Geometry check sheet. Reference: the model listing, model coordinates, mm. Face numbers are marked on the shaded views. A direction names the side the tool comes from. Give positions to 0.01 mm unless a question says otherwise; leave off trailing zeros. Order: outer loops, then holes, each group sorted by start corner. A loop starts at its lowest first (then second) coordinate and runs counter-clockwise, first axis right, second up. Notation, with made-up numbers: M -17,84.5 L -5,84.5 A22 ccw -5,107.5 Z; hole C 84.25,46.25 d1. An arc over 180 degrees is marked long. One line per question, with ' | ' between items. Start each with the question number.
from build123d import *
from OCP.BRepFilletAPI import BRepFilletAPI_MakeChamfer

# Parameters (mm, degrees)
SKETCH1_W           = 1.85
SKETCH1_H           = 38.85
SKETCH1_H_2         = 6.15
SKETCH1_W_2         = 44.85
SKETCH1_H_3         = 1.85
SKETCH1_W_3         = 0.15
BOSS_EXTRUDE1_DEPTH = 3
SKETCH1_4_W         = 120
SKETCH1_4_H         = 30
SKETCH1_4_W_2       = 30
SKETCH1_4_H_2       = 120
BOSS_EXTRUDE3_DEPTH = 4
CHAMFER1_SIZE       = 2.5
CHAMFER1_SIZE2      = 9.330127019
SKETCH4_W           = 8.5
SKETCH4_H           = 30
SKETCH4_W_2         = 30
SKETCH4_H_2         = 8.5
CUT_EXTRUDE1_DEPTH  = 1.5
BOSS_EXTRUDE4_DEPTH = 35
CHAMFER2_SIZE       = 6
BOSS_EXTRUDE5_DEPTH = 3
CHAMFER3_SIZE       = 2
CHAMFER3_SIZE2      = 5.494954839
BOSS_EXTRUDE6_DEPTH = 2.5


with BuildPart() as part:
    # Sketch1 → Boss-Extrude1 (new body)
    with BuildSketch(Plane(origin=(0, 0, 0), x_dir=(-1, 0, 0), z_dir=(0, 0, -1))):
        with Locations((14.075, 40.575)):
            Rectangle(SKETCH1_W, SKETCH1_H)
        with Locations((14.075, 18.075)):
            Rectangle(SKETCH1_W, SKETCH1_H_2)
        with Locations((37.575, 14.075)):
            Rectangle(SKETCH1_W_2, SKETCH1_H_3)
        with Locations((14.075, 14.075)):
            Rectangle(SKETCH1_W, SKETCH1_H_3)
        with Locations((14.075, -14.075)):
            Rectangle(SKETCH1_W, SKETCH1_H_3)
        with Locations((14.075, -18.075)):
            Rectangle(SKETCH1_W, SKETCH1_H_2)
        with Locations((37.575, -14.075)):
            Rectangle(SKETCH1_W_2, SKETCH1_H_3)
        with Locations((14.075, -40.575)):
            Rectangle(SKETCH1_W, SKETCH1_H)
        with Locations((-14.075, -14.075)):
            Rectangle(SKETCH1_W, SKETCH1_H_3)
        with Locations((-14.075, -18.075)):
            Rectangle(SKETCH1_W, SKETCH1_H_2)
        with Locations((-37.575, -14.075)):
            Rectangle(SKETCH1_W_2, SKETCH1_H_3)
        with Locations((-15.075, -14.075)):
            Rectangle(SKETCH1_W_3, SKETCH1_H_3)
        with Locations((15.075, -14.075)):
            Rectangle(SKETCH1_W_3, SKETCH1_H_3)
        with Locations((15.075, 14.075)):
            Rectangle(SKETCH1_W_3, SKETCH1_H_3)
        with Locations((-37.575, 14.075)):
            Rectangle(SKETCH1_W_2, SKETCH1_H_3)
        with Locations((-15.075, 14.075)):
            Rectangle(SKETCH1_W_3, SKETCH1_H_3)
        with Locations((-14.075, 18.075)):
            Rectangle(SKETCH1_W, SKETCH1_H_2)
        with Locations((-14.075, 14.075)):
            Rectangle(SKETCH1_W, SKETCH1_H_3)
        with Locations((-14.075, 40.575)):
            Rectangle(SKETCH1_W, SKETCH1_H)
        with Locations((-14.075, -40.575)):
            Rectangle(SKETCH1_W, SKETCH1_H)
    extrude(amount=-BOSS_EXTRUDE1_DEPTH)

    # Sketch1<4> → Boss-Extrude3 (add)
    with BuildSketch(Plane(origin=(0, 0, 0), x_dir=(-1, 0, 0), z_dir=(0, 0, -1))):
        Rectangle(SKETCH1_4_W, SKETCH1_4_H)
        Rectangle(SKETCH1_4_W_2, SKETCH1_4_H_2)
    extrude(amount=BOSS_EXTRUDE3_DEPTH)

    # Chamfer1: one chamfer whose edges measure the first distance from different faces: ONE call of the kernel's chamfer builder (chamfer() names one face for all edges)
    chamfer1_edges_1 = [part.edges().sort_by_distance(p)[0] for p in [
        (60, 0, -4),
    ]]
    chamfer1_side_1 = [part.faces().sort_by_distance(p)[0] for p in [
        (60, 0, -1.703661327),
    ]]
    chamfer1_edges_2 = [part.edges().sort_by_distance(p)[0] for p in [
        (0, 60, -4),
    ]]
    chamfer1_side_2 = [part.faces().sort_by_distance(p)[0] for p in [
        (0, 60, -1.703661327),
    ]]
    chamfer1_edges_3 = [part.edges().sort_by_distance(p)[0] for p in [
        (0, -60, -4),
    ]]
    chamfer1_side_3 = [part.faces().sort_by_distance(p)[0] for p in [
        (0, -60, -1.703661327),
    ]]
    chamfer1_edges_4 = [part.edges().sort_by_distance(p)[0] for p in [
        (-60, 0, -4),
    ]]
    chamfer1_side_4 = [part.faces().sort_by_distance(p)[0] for p in [
        (-60, 0, -1.703661327),
    ]]
    chamfer1 = BRepFilletAPI_MakeChamfer(part.part.solid().wrapped)
    for e in chamfer1_edges_1:
        chamfer1.Add(CHAMFER1_SIZE, CHAMFER1_SIZE2, e.wrapped, chamfer1_side_1[0].wrapped)  # the first distance lies on this face
    for e in chamfer1_edges_2:
        chamfer1.Add(CHAMFER1_SIZE, CHAMFER1_SIZE2, e.wrapped, chamfer1_side_2[0].wrapped)  # the first distance lies on this face
    for e in chamfer1_edges_3:
        chamfer1.Add(CHAMFER1_SIZE, CHAMFER1_SIZE2, e.wrapped, chamfer1_side_3[0].wrapped)  # the first distance lies on this face
    for e in chamfer1_edges_4:
        chamfer1.Add(CHAMFER1_SIZE, CHAMFER1_SIZE2, e.wrapped, chamfer1_side_4[0].wrapped)  # the first distance lies on this face
    add(Compound.cast(chamfer1.Shape()), mode=Mode.REPLACE)

    # Sketch4 → Cut-Extrude1 (cut)
    with BuildSketch(Plane(origin=(0, 0, -4), x_dir=(-1, 0, 0), z_dir=(0, 0, -1))):
        with Locations((-41.419872981, 0)):
            Rectangle(SKETCH4_W, SKETCH4_H)
        with Locations((-29.919872981, 0)):
            Rectangle(SKETCH4_W, SKETCH4_H)
        with Locations((0, 41.419872981)):
            Rectangle(SKETCH4_W_2, SKETCH4_H_2)
        with Locations((0, 29.919872981)):
            Rectangle(SKETCH4_W_2, SKETCH4_H_2)
        with Locations((29.919872981, 0)):
            Rectangle(SKETCH4_W, SKETCH4_H)
        with Locations((41.419872981, 0)):
            Rectangle(SKETCH4_W, SKETCH4_H)
        with Locations((0, -29.919872981)):
            Rectangle(SKETCH4_W_2, SKETCH4_H_2)
        with Locations((0, -41.419872981)):
            Rectangle(SKETCH4_W_2, SKETCH4_H_2)
    extrude(amount=-CUT_EXTRUDE1_DEPTH, mode=Mode.SUBTRACT)

    # Sketch5 → Boss-Extrude4 (add)
    with BuildSketch(Plane(origin=(0, 0, -4), x_dir=(-1, 0, 0), z_dir=(0, 0, -1))):
        Polygon((-7.424621202, 3.181980515), (-3.181980515, 7.424621202), (7.424621202, -3.181980515), (3.181980515, -7.424621202), align=None)
    extrude(amount=BOSS_EXTRUDE4_DEPTH)

    # Chamfer2
    chamfer2_edges = [part.edges().sort_by_distance(p)[0] for p in [
        (-2.121320344, 2.121320344, -39),
    ]]
    chamfer(chamfer2_edges, length=CHAMFER2_SIZE - 0.0001)  # a hair under: the kernel refuses the full size

    # Sketch6 → Boss-Extrude5 (add)
    with BuildSketch(Plane(origin=(-12.727922061, 12.727922061, -18), x_dir=(-0.8660254037844379, -0.28867513459481464, 0.4082482904638634), z_dir=(-0.5000000000000013, 0.5000000000000013, -0.7071067811865458))):
        Polygon((-23.270152556, -19.918584287), (-11.723147173, -3.588652668), (0.524301541, -12.248906706), (-11.022703843, -28.578838325), align=None)
    extrude(amount=BOSS_EXTRUDE5_DEPTH)

    # Chamfer3
    chamfer3_edges = [part.edges().sort_by_distance(p)[0] for p in [
        (-9.378679656, 9.378679656, -26.97918472),
    ]]
    chamfer3_side = [part.faces().sort_by_distance(p)[0] for p in [
        (-8.628679656, 8.628679656, -25.918524548),
    ]]
    chamfer(chamfer3_edges, length=CHAMFER3_SIZE, length2=CHAMFER3_SIZE2, reference=chamfer3_side[0])

    # Sketch8 → Boss-Extrude6 (add)
    with BuildSketch(Plane(origin=(-11.477922061, 11.477922061, -16.232233047), x_dir=(0.8660254037844378, 0.28867513459481475, -0.4082482904638635), z_dir=(0.5000000000000016, -0.5000000000000013, 0.7071067811865456))):
        Polygon((6.123724357, -21.650635095), (18.371173071, -12.990381057), (9.885891697, -0.990381057), (-2.361557017, -9.650635095), align=None)
    extrude(amount=BOSS_EXTRUDE6_DEPTH)


solid = part.part
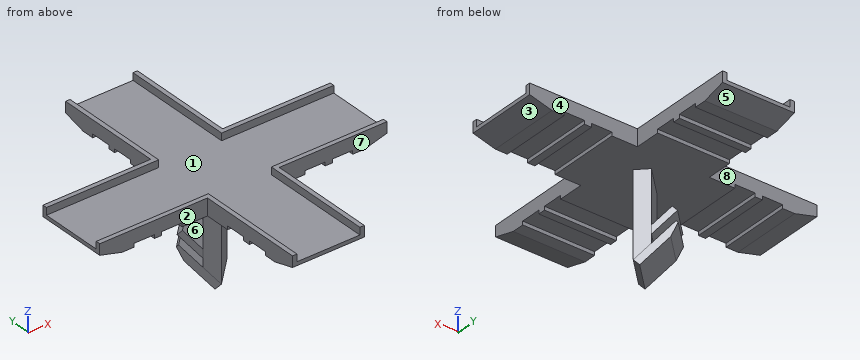
Item 1: Cross-section at B-B, the plane y = 22.5. Record the cut outline in (x, z), plus the area to 3 significant figures.
Item 2: Depth check by flat-ended pin: pin 1 (2 mm diameter, centred on x = -7.5, z = -8.5, fed in from -Y); pin 2 (0.9 mm diameter, centred on y = 44.5, z = 1, fed in from -X); pin 3 (2 mm diameter, centred on x = -32.5, z = 0, fed in from -Y). Enter the tip coordinate at first touch or a pass-through.
Item 3: Mould release check, pull along X, two halves, no side actions. Record for the marked faces 1, 2 and 3: released by +X, released by -X, zero draft, split by the parting line, or undercut.
Item 4: Set-up check for the marked faces 4, 5, 6, 7 and 8: record each of +Z, -Z, +X, -X, +Y, -Y from which the full face is reachable in a straight line by a thin tool's end or side.
Item 5: Cross-section at A-A, the plane x = -30. Record the cut outline in (y, z), plus the area to 3 significant figures.
Item 6: Material ranges on line 1 along X through (y, z) = (19, 0.5); line 2 along X through (y, z) = (-19, -0.5); line 3 along Z through (x, y) = (0, -44.5), recorded low to high.
Item 7: Cross-section at C-C, the plane z = -15. Record the cut outline in (x, y), plus the area to 3 significant figures.
Item 8: Cross-section at D-D, the plane z = -37.5. Record the cut outline in (x, y).
Outcome:
1) outline: M -15,-4 L 15,-4 L 15,3 L 13.15,3 L 13.15,0 L -13.15,0 L -13.15,3 L -15,3 Z | area: 131 mm²
2) pin 1: stops at y = -4.11 | pin 2: stops at x = -15 | pin 3: stops at y = -15
3) face 1: undercut | face 2: zero draft | face 3: released by +X
4) face 4: +Z, -Z, +X, +Y | face 5: -Z, +X, -X, +Y | face 6: none | face 7: +Z, -Z, +X, -Y | face 8: +Z, -Z, -X, +Y
5) outline: M -15,-2.5 L 15,-2.5 L 15,3 L 13.15,3 L 13.15,0 L -13.15,0 L -13.15,3 L -15,3 Z | area: 86.1 mm²
6) line 1: x = -15 to -13.15, 13.15 to 15 | line 2: x = -15 to 15 | line 3: z = -2.5 to 0
7) outline: M -7.42,-3.18 L -3.18,-7.42 L 7.42,3.18 L 3.18,7.42 Z | area: 90.0 mm²
8) outline: M -7.24,-3.36 L -3.18,-7.42 L 7.42,3.18 L 3.36,7.24 Z
